```python
from build123d import *

# Parameters (mm, degrees)
SKETCH_1_R          = 12.5
EXTRUDE_1_DEPTH     = 17.5
SKETCH_2_R          = 9
EXTRUDE_2_DEPTH     = 55
SKETCH_3_R          = 6
EXTRUDE_3_DEPTH     = 10
CHAMFER_1_SIZE      = 0.5
SKETCH_4_R          = 5
CUT_EXTRUDE_1_DEPTH = 139
CHAMFER_2_SIZE      = 1
SKETCH_5_R          = 8
CUT_EXTRUDE_2_DEPTH = 12


with BuildPart() as part:
    # 草图1 → 凸台-拉伸1 (new body)
    with BuildSketch(Plane.XY):
        Circle(SKETCH_1_R)
    extrude(amount=EXTRUDE_1_DEPTH)

    # 草图2 → 凸台-拉伸2 (add)
    with BuildSketch(Plane(origin=(0, 0, 0), x_dir=(-1, 0, 0), z_dir=(0, 0, -1))):
        Circle(SKETCH_2_R)
    extrude(amount=EXTRUDE_2_DEPTH)

    # 草图3 → 凸台-拉伸3 (add)
    with BuildSketch(Plane(origin=(0, 0, -55), x_dir=(-1, 0, 0), z_dir=(0, 0, -1))):
        Circle(SKETCH_3_R)
    extrude(amount=EXTRUDE_3_DEPTH)

    # 倒角1
    chamfer_1_edges = [part.edges().sort_by_distance(p)[0] for p in [
        (6, 0, -65),
    ]]
    chamfer(chamfer_1_edges, length=CHAMFER_1_SIZE)

    # 草图4 → 切除-拉伸1 (cut)
    with BuildSketch(Plane(origin=(0, 0, -65), x_dir=(-1, 0, 0), z_dir=(0, 0, -1))):
        Circle(SKETCH_4_R)
    extrude(amount=-CUT_EXTRUDE_1_DEPTH, mode=Mode.SUBTRACT)

    # 倒角2
    chamfer_2_edges = [part.edges().sort_by_distance(p)[0] for p in [
        (9, 0, -55),
    ]]
    chamfer(chamfer_2_edges, length=CHAMFER_2_SIZE)

    # 草图5 → 切除-拉伸2 (cut)
    with BuildSketch(Plane.XY.offset(17.5)):
        Circle(SKETCH_5_R)
    extrude(amount=-CUT_EXTRUDE_2_DEPTH, mode=Mode.SUBTRACT)


solid = part.part
```
The model under review builds one solid part; all positions refer to its coordinate system, in mm. A direction names the side the tool comes from. Round coordinates to 2 decimals unless told otherwise and drop trailing zeros. Loops run counter-clockwise (first coordinate to the right, second up) from the corner with the lowest first, then second, coordinate; pieces in that order, holes last. Notation, with made-up numbers: (27, 80.25) - (38, 80.25) arc R18 ccw to (38, 90.25) - close; hole circle Ø9 at (-31.75, 39.25). An arc over 180 degrees is marked (long way). Use a Markdown table: item, result. Add a question column.
Q1. Insertion check: pin 1 Ø3 at (x, y) = (-4.5, -5.5) entering from -Z; pin 2 Ø6 at (x, z) = (-9.5, -45.5) entering from -Y; pin 3 Ø11.5 at (x, y) = (0, 0) entering from +Z; pin 4 Ø5 at (x, y) = (2, 4) entering from -Z. Each pin has a flat end and moves straight along its axis. Give the tip position at first contact, or say it passes through.
Q2. Add section A-A (y = 0). State the section outline as (x, z) points, plus the area to 3 significant figures.
Q3. Add section C-C (z = -2). State the section outline as (x, y) points.
Q4. For probe 1 along Y at (x, z) = (0, 14.5); probe 2 along Y at (x, z) = (0, -45.5); probe 3 along Z at (x, y) = (6.75, 4), list the stretches that pass through material, from the lowest coordinate up.
Q5. The part is to be moulded in two halves that separate along X. For faces 1 (the face through (1.08, -4.88, -30.24)), 2 (the face through (-1.6, -4.9, -65)), 3 (the face through (11.923, 3.755, 8.628)), say which applies: pulls with the +X half, pulls with the -X half, needs draft (parallel to the pull), parting line crosses it, or undercut.
Q6. Machinability: for faces 4 (the face through (1.172, 8.923, -26.622)), 5 (the face through (-0.2, -8.2, 17.5)), 6 (the face through (5.2, 0.1, 5.5)), which of the approach directions +Z, -Z, +X, -X, +Y, -Y give a long, thin tool a straight path to every point of the face, cutting with its end or side? Answer none if there is none.
Worked answers:
| question | item | result |
|---|---|---|
| 1 | pin 1 | z = -64.89 |
| 1 | pin 2 | y = -6.22 |
| 1 | pin 3 | z = 5.5 |
| 1 | pin 4 | z = -65 |
| 2 | outline | (-12.5, 0) - (-9, 0) - (-9, -54) - (-8, -55) - (-6, -55) - (-6, -64.5) - (-5.5, -65) - (-5, -65) - (-5, 5.5) - (-8, 5.5) - (-8, 17.5) - (-12.5, 17.5) - close; (5, -65) - (5.5, -65) - (6, -64.5) - (6, -55) - (8, -55) - (9, -54) - (9, 0) - (12.5, 0) - (12.5, 17.5) - (8, 17.5) - (8, 5.5) - (5, 5.5) - close |
| 2 | area | 649 mm² |
| 3 | outline | circle Ø18 at (0, 0); hole circle Ø10 at (0, 0) |
| 4 | probe 1 | -12.5 to -8, 8 to 12.5 |
| 4 | probe 2 | -9 to -5, 5 to 9 |
| 4 | probe 3 | -55 to 5.5 |
| 5 | face 1 | undercut |
| 5 | face 2 | needs draft |
| 5 | face 3 | parting line crosses it |
| 6 | face 4 | -Z |
| 6 | face 5 | +Z, +X, -X, +Y, -Y |
| 6 | face 6 | +Z |
